Model file for the job. Use its own axes, mm. A direction names the side the tool comes from. Round coordinates to 2 decimals unless told otherwise and drop trailing zeros. Order: outer loops, then holes, each group sorted by start corner. A loop starts at its lowest first (then second) coordinate and runs counter-clockwise, first axis right, second up. Notation, with made-up numbers: (64, 8) - (81, 8) arc R28 ccw to (81, 36) - close; hole circle Ø6 at (58.5, 76). An arc over 180 degrees is marked (long way). Write item = value, one per line.
```python
from build123d import *

# Parameters (mm, degrees)
SKETCH1_R           = 2.075
BOSS_EXTRUDE1_DEPTH = 1
FILLET1_R           = 2


with BuildPart() as part:
    # Sketch1 → Boss-Extrude1 (new, symmetric)
    with BuildSketch(Plane.XY):
        with BuildLine():
            Line((-10.075, 76.2), (-10.075, 0))
            ThreePointArc((-10.075, 0), (-7.12410082, -7.12410082), (0, -10.075))
            Line((0, -10.075), (50.8, -10.075))
            ThreePointArc((50.8, -10.075), (60.875, 0), (50.8, 10.075))
            Line((50.8, 10.075), (10.075, 10.075))
            Line((10.075, 10.075), (10.075, 76.2))
            ThreePointArc((10.075, 76.2), (0, 86.275), (-10.075, 76.2))
        make_face()
        Circle(SKETCH1_R, mode=Mode.SUBTRACT)
        with Locations((12.7, 0)):
            Circle(SKETCH1_R, mode=Mode.SUBTRACT)
        with Locations((25.4, 0)):
            Circle(SKETCH1_R, mode=Mode.SUBTRACT)
        with Locations((38.1, 0)):
            Circle(SKETCH1_R, mode=Mode.SUBTRACT)
        with Locations((50.8, 0)):
            Circle(SKETCH1_R, mode=Mode.SUBTRACT)
        with Locations((0, 12.7)):
            Circle(SKETCH1_R, mode=Mode.SUBTRACT)
        with Locations((0, 25.4)):
            Circle(SKETCH1_R, mode=Mode.SUBTRACT)
        with Locations((0, 38.1)):
            Circle(SKETCH1_R, mode=Mode.SUBTRACT)
        with Locations((0, 50.8)):
            Circle(SKETCH1_R, mode=Mode.SUBTRACT)
        with Locations((0, 63.5)):
            Circle(SKETCH1_R, mode=Mode.SUBTRACT)
        with Locations((0, 76.2)):
            Circle(SKETCH1_R, mode=Mode.SUBTRACT)
    extrude(amount=BOSS_EXTRUDE1_DEPTH, both=True)

    # Fillet1
    fillet1_edges = [part.edges().sort_by_distance(p)[0] for p in [
        (10.075, 10.075, 0),
    ]]
    fillet(fillet1_edges, radius=FILLET1_R)


solid = part.part
```
1) Cut at B-B (z = -0.3). Give the number of separate pieces and of enclosed holes in the cut face, and give its area (3 significant figures).
Conclusion:
separate_pieces = 1
enclosed_holes = 11
area = 2,710 mm^2
2) Wall check: line 1 along X through (y, z) = (76.5, 0.9); line 2 along X through (y, z) = (0.5, 0) (3 decimals); line 3 along Y through (x, z) = (12.7, 0.3) (3 decimals). Give the ranges that are in metal, low to high.
Conclusion:
line_1 = -10.07 to -2.05, 2.05 to 10.07
line_2 = -10.075 to -2.014, 2.014 to 10.686, 14.714 to 23.386, 27.414 to 36.086, 40.114 to 48.786, 52.814 to 60.863
line_3 = -10.075 to -2.075, 2.075 to 10.075
3) Cut at C-C (y = 33). Write the cut outline in (x, z) (3 decimals).
Conclusion:
outline = (-10.075, -1) - (10.075, -1) - (10.075, 1) - (-10.075, 1) - close
4) 3-axis set-ups, long thin cutter, end or side, ignore diameter. For faces 1 (the face through (32, 10.075, 0)), 2 (the face through (1.116, 27.15, -0.014)): which of +Z, -Z, +X, -X, +Y, -Y reach the whole face in a straight line?
Conclusion:
face_1 = +Z, -Z, +X, +Y
face_2 = +Z, -Z
5) Cut at A-A (x = 25.4). Write the cut outline in (y, z) (3 decimals).
Conclusion:
outline = (-10.075, -1) - (-2.075, -1) - (-2.075, 1) - (-10.075, 1) - close; (2.075, -1) - (10.075, -1) - (10.075, 1) - (2.075, 1) - close
6) Flat gauge pins, fed straight in: pin 1 Ø1 at (x, z) = (6.5, -0.5) entering from +Y; pin 2 Ø1 at (y, z) = (6, 0) entering from +X; pin 3 Ø0.6 at (x, z) = (37.5, 0) entering from +Y (3 decimals). Where does each tip first touch, or does it go through?
Conclusion:
pin_1 = 84.29
pin_2 = 59.24
pin_3 = 10.075
